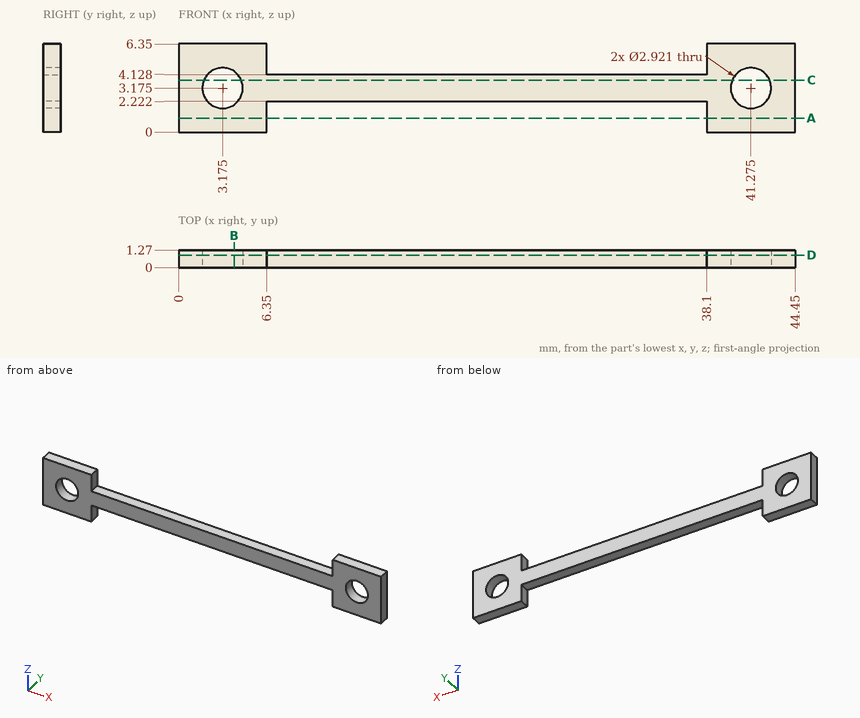
Here's the drawing with two shaded views (mm, measured from the low corner). I have some questions. Give positions to 0.01 mm unless a question says otherwise; leave off trailing zeros. Write each loop counter-clockwise with the first axis right and the second up, starting at its lowest first coordinate (ties: lowest second). Pieces come first, ordered by that corner, then holes. Notation, with made-up numbers: (-40, 12.5) -> (6, 12.5) arc R14 cw to (6, 29.5) -> close; hole circle Ø10 at (-12.75, 16.25). An arc over 180 degrees is marked (long way). Answer as a JSON object with one key per item and string values. Group by question number.
Item 1: Suppose I cut it at B-B (x = 4). Please give me the cut outline in (y, z).
Item 2: Suppose I cut it at D-D (y = 0.9). State how many separate pieces and enclosed holes the cut face has, plus the area to 3 significant figures.
Item 3: I'm going to push a flat-ended pin straight in: P1, Ø0.6, axis at x = 24, y = 0.5, coming from the -Z side. Where does the tip first touch, or does it pass through?
Item 4: Please list where these lines run through material, in increasing order: line 1 (X direction, y = 0.9, z = 3.75); line 2 (X direction, y = 0.8, z = 5.75); line 3 (X direction, y = 0.55, z = 3.5). Write a range as [from, to].
Item 5: Suppose I cut it at A-A (z = 1). Please give me the cut outline in (x, y).
Item 6: Suppose I cut it at C-C (z = 3.75). Please give me the cut outline in (x, y).
Findings:
{
 "1": {"outline": "(0, 0) -> (1.27, 0) -> (1.27, 1.97) -> (0, 1.97) -> close; (0, 4.38) -> (1.27, 4.38) -> (1.27, 6.35) -> (0, 6.35) -> close"},
 "2": {"separate pieces": "1", "enclosed holes": "2", "area": "128 mm²"},
 "3": {"P1": "stops at z = 2.22"},
 "4": {"line 1": "x = [0, 1.83], [4.52, 39.93], [42.62, 44.45]", "line 2": "x = [0, 6.35], [38.1, 44.45]", "line 3": "x = [0, 1.75], [4.6, 39.85], [42.7, 44.45]"},
 "5": {"outline": "(0, 0) -> (6.35, 0) -> (6.35, 1.27) -> (0, 1.27) -> close; (38.1, 0) -> (44.45, 0) -> (44.45, 1.27) -> (38.1, 1.27) -> close"},
 "6": {"outline": "(0, 0) -> (1.83, 0) -> (1.83, 1.27) -> (0, 1.27) -> close; (4.52, 0) -> (39.93, 0) -> (39.93, 1.27) -> (4.52, 1.27) -> close; (42.62, 0) -> (44.45, 0) -> (44.45, 1.27) -> (42.62, 1.27) -> close"}
}
